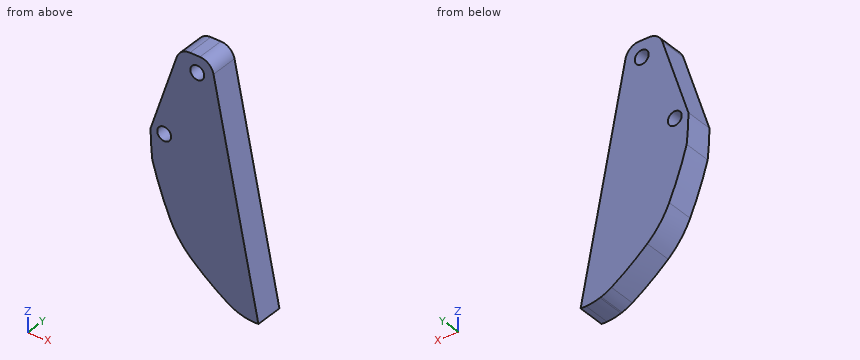
from build123d import *

# Parameters (mm, degrees)
SKETCH2_R           = 1
BOSS_EXTRUDE2_DEPTH = 4
FILLET1_R           = 13
FILLET2_R           = 7
FILLET4_R           = 7


with BuildPart() as part:
    # Sketch2 → Boss-Extrude2 (new body)
    with BuildSketch(Plane(origin=(0, 0, 0), x_dir=(1, 0, 0), z_dir=(0, 1, 0))):
        with BuildLine():
            Line((-5.254491041, 13.546811275), (-1.48741211, 2.139537078))
            ThreePointArc((-1.48741211, 2.139537078), (-0.759971379, 1.145843389), (0.411712444, 0.766694098))
            Line((0.411712444, 0.766694098), (1.855419889, 0.766694098))
            ThreePointArc((1.855419889, 0.766694098), (3.121752187, 1.218662279), (3.815742579, 2.370291586))
            Line((3.815742579, 2.370291586), (10.286953209, 34.372260906))
            ThreePointArc((10.286953209, 34.372260906), (9.271638883, 34.372242241), (8.262186146, 34.263300263))
            ThreePointArc((8.262186146, 34.263300263), (7.370397326, 33.984118682), (6.494594719, 33.658236114))
            ThreePointArc((6.494594719, 33.658236114), (2.361803433, 30.744474886), (-1.353992878, 27.314777221))
            ThreePointArc((-1.353992878, 27.314777221), (-3.406730235, 22.664628668), (-5.003894853, 17.839001517))
            ThreePointArc((-5.003894853, 17.839001517), (-5.179724164, 15.695856621), (-5.254491041, 13.546811275))
        make_face()
        with Locations(Location((1.478658486, 3.11569661, 0), (0, 0, 270))):
            Circle(SKETCH2_R, mode=Mode.SUBTRACT)
        with Locations(Location((-3.294171009, 13.546811275, 0), (0, 0, 270))):
            Circle(SKETCH2_R, mode=Mode.SUBTRACT)
        with BuildLine():
            ThreePointArc((-1.76086985, 10.970987524), (-1.889568474, 10.993883735), (-2.020154104, 10.999796885))
            ThreePointArc((-2.020154104, 10.999796885), (-1.890628473, 10.984343745), (-1.76086985, 10.970987524))
        make_face(mode=Mode.SUBTRACT)
    extrude(amount=BOSS_EXTRUDE2_DEPTH)

    # Fillet1
    fillet1_edges = [part.edges().sort_by_distance(p)[0] for p in [
        (-1.353992878, 2, -27.314777221),
    ]]
    fillet(fillet1_edges, radius=FILLET1_R)

    # Fillet2
    fillet2_edges = [part.edges().sort_by_distance(p)[0] for p in [
        (8.262186146, 2, -34.263300263),
    ]]
    fillet(fillet2_edges, radius=FILLET2_R)

    # Fillet4
    fillet4_edges = [part.edges().sort_by_distance(p)[0] for p in [
        (6.494594719, 2, -33.658236114),
    ]]
    fillet(fillet4_edges, radius=FILLET4_R)


solid = part.part
The model under review builds one solid part; all positions refer to its coordinate system, in mm. Give positions to 0.01 mm unless a question says otherwise; leave off trailing zeros. Loops run counter-clockwise (first coordinate to the right, second up) from the corner with the lowest first, then second, coordinate; pieces in that order, holes last. Notation, with made-up numbers: (31, -16) -> (54, -16) arc R31 ccw to (54, 10) -> close; hole circle Ø5 at (-12, 31). An arc over 180 degrees is marked (long way). Answer as a JSON object with one key per item and string values. Group by question number.
Q1. Wall thickness on line 1 along Z through (x, y) = (1.5, 2.75); line 2 along X through (y, z) = (2.75, -26.5); line 3 along X through (y, z) = (0.5, -28.5): over which ranges is each line inside the solid? List them lowest first.
Q2. Take a section at B-B (y = 2.35). State how many separate pieces and enclosed holes the cut face has, plus the area to 3 significant figures.
Q3. Take a section at C-C (x = 5.5). Write out the cut boundary in (y, z), plus the area to 3 significant figures.
Q4. Insertion check: pin 1 (3 mm diameter, centred on x = 7, z = -30.5, fed in from -Y); pin 2 (2 mm diameter, centred on y = 3.5, z = -21.5, fed in from +X); pin 3 (1 mm diameter, centred on y = 1.5, z = -26.5, fed in from -X). Each pin has a flat end and moves straight along its axis. Give the tip position at first contact, or say it passes through.
Q5. Take a section at A-A (z = -22.5). Write out the cut boundary in (x, y).
Answer below:
{
 "1": {"line 1": "z = -30.03 to -4.12, -2.12 to -0.77", "line 2": "x = -1.65 to 8.7", "line 3": "x = -0.13 to 9.1"},
 "2": {"separate pieces": "1", "enclosed holes": "3", "area": "299 mm2"},
 "3": {"outline": "(0, -33.03) -> (4, -33.03) -> (4, -10.7) -> (0, -10.7) -> close", "area": "89.3 mm2"},
 "4": {"pin 1": "stops at y = 0", "pin 2": "stops at x = 7.89", "pin 3": "stops at x = -1.94"},
 "5": {"outline": "(-3.47, 0) -> (7.89, 0) -> (7.89, 4) -> (-3.47, 4) -> close"}
}
